from build123d import *

# Parameters (mm, degrees)
SKETCH_R      = 7.5
SKETCH_R_2    = 6
PAD_DEPTH     = 4
SKETCH001_R   = 7.5
SKETCH001_R_2 = 1.6
PAD001_DEPTH  = 2
FILLET_R      = 0.99


with BuildPart() as part:
    # Sketch → Pad (new body)
    with BuildSketch(Plane.XY):
        Circle(SKETCH_R)
        Circle(SKETCH_R_2, mode=Mode.SUBTRACT)
    extrude(amount=-PAD_DEPTH)

    # Sketch001 → Pad001 (join)
    with BuildSketch(Plane.XY):
        Circle(SKETCH001_R)
        Circle(SKETCH001_R_2, mode=Mode.SUBTRACT)
    extrude(amount=PAD001_DEPTH)

    # Fillet
    fillet_edges = [part.edges().sort_by_distance(p)[0] for p in [
        (-1.6, 0, 2),
        (-1.6, 0, 0),
        (-7.5, 0, 2),
        (-6, 0, -4),
    ]]
    fillet(fillet_edges, radius=FILLET_R)


solid = part.part
Read the model definition and answer for the solid it produces. Units are mm, in the model's axes. Coordinates: 2 decimals unless noted, no trailing zeros. Loops run counter-clockwise (first coordinate to the right, second up) from the corner with the lowest first, then second, coordinate; pieces in that order, holes last. Notation, with made-up numbers: (-37.5, 52.25) - (-13.5, 52.25) arc R30 cw to (-13.5, 84.25) - close; hole circle Ø6 at (-5, 18). An arc over 180 degrees is marked (long way). Answer in a Markdown table with one row per item.
Q1. Find section D-D on z = 0.5. Write down the section's boundary in (x, y).
Here are the results:
| item | result |
|---|---|
| outline | circle Ø15 at (0, 0); hole circle Ø3.46 at (0, 0) |
Q2. Given P1, Ø1.5, axis at y = -2.5, z = -2, coming from the +X side; P2, Ø5, axis at x = 0, y = 0, coming from the +Z side; P3, Ø3.5, axis at x = 2, y = 2, coming from the -Z side, each flat-ended and moving along its own axis, determine where each tip first touches the part or whether it passes through.
Here are the results:
| item | result |
|---|---|
| P1 | stops at x = 7.29 |
| P2 | stops at z = 2 |
| P3 | stops at z = 0 |
Q3. Find section C-C on z = -2.35. Write down the section's boundary in (x, y).
Here are the results:
| item | result |
|---|---|
| outline | circle Ø15 at (0, 0); hole circle Ø12 at (0, 0) |
Q4. The mould has two halves that part along X. Classify faces 1 (the cylindrical face through (-6, 0, -1)), 2 (the flat face through (3, -1, 0)), 3 (the flat face through (3, 0, 2)): pulls with the +X half, pulls with the -X half, needs draft (parallel to the pull), parting line crosses it, or undercut.
Here are the results:
| item | result |
|---|---|
| face 1 | undercut |
| face 2 | undercut |
| face 3 | needs draft |
Q5. Straight lines are drawn through the part: line 1 along Y through (x, z) = (0, -0.75); line 2 along Y through (x, z) = (0, 1); line 3 along Z through (x, y) = (3.75, 2). For each, find the intervals that lie inside material, in ascending order. Write a range as [from, to].
Here are the results:
| item | result |
|---|---|
| line 1 | y = [-7.5, -6], [6, 7.5] |
| line 2 | y = [-7.5, -1.6], [1.6, 7.5] |
| line 3 | z = [0, 2] |
